Check sheet for the modelled part. Datum: model origin and axes. Units: mm. Give positions to 0.01 mm unless a question says otherwise; leave off trailing zeros. Loops run counter-clockwise (first coordinate to the right, second up) from the corner with the lowest first, then second, coordinate; pieces in that order, holes last. Notation, with made-up numbers: (78, 73.5) -> (127, 73.5) arc R5 ccw to (127, 80.5) -> close; hole circle Ø2 at (44, 33). An arc over 180 degrees is marked (long way). Write each question's results on one line, items separated by ' | '. Start each with the question number.
Item 1: Cross-section at D-D on z = 0.75. Enter the section's corners in (x, y), then the cut area to 3 significant figures.
Item 2: Mould release check, pull along X, two halves, no side actions. Record for faces 1 (the face through (17.5, 0, 0)), 2 (the face through (12.43, -3.905, 0.867)), 3 (the face through (-9.87, 1.6, 0.22)), 4 (the face through (1.09, -0.05, -4.88)): pulls with the +X half, pulls with the -X half, needs draft (parallel to the pull), parting line crosses it, or undercut.
Item 3: Cross-section at B-B on x = 15.25. Enter the section's corners in (y, z), then the cut area to 3 significant figures.
Item 4: Scan lines: line 1 along X through (y, z) = (-5, 0.5); line 2 along X through (y, z) = (7.5, 4); line 3 along Z through (x, y) = (2.5, 6.5). Record each from-to range of solid material in increasing order.
Item 5: Gauge pin test, flat ends, axial feed: pin 1 Ø12 at (x, z) = (8.5, -4) entering from +Y; pin 2 Ø2 at (y, z) = (8.5, 3.5) entering from +X; pin 3 Ø5 at (x, z) = (-7.5, 0) entering from -Y; pin 4 Ø12 at (y, z) = (6, 3.5) entering from +X. Record the tip position at first contact, or that the pin passes through.
Item 6: Cross-section at C-C on z = -5.5. Enter the section's corners in (x, y).
Item 7: Cross-section at A-A on z = -3. Enter the section's corners in (x, y).
from build123d import *

# Parameters (mm, degrees)
EXTRUDE_3_DEPTH      = 10
EXTRUDE_3_DEPTH_BACK = 10
SKETCH_3_R           = 5
CUT_EXTRUDE_1_DEPTH  = 27.477518989
EXTRUDE_6_DEPTH      = 10
EXTRUDE_6_DEPTH_BACK = 10
SKETCH_9_R           = 4
EXTRUDE_8_DEPTH      = 10


with BuildPart() as part:
    # Sketch 3D_4 → Extrude 3 (new, two sides: drawn at the far end of the back side and taken through both)
    with BuildSketch(Plane(origin=(0, 0, -10), x_dir=(0.24333901077648587, -0.042907233058801585, 0.9689917931466494), z_dir=(0.17364817766692725, 0.9848077530122086, 0)).offset(-EXTRUDE_3_DEPTH_BACK)):
        with BuildLine():
            Line((0, 0), (1.260173827, 4.941858145))
            Line((1.260173827, 4.941858145), (20.64000969, 0))
            Line((20.64000969, 0), (19.379835863, -4.941858145))
            ThreePointArc((19.379835863, -4.941858145), (7.218988859, -12.160847004), (0, 0))
        make_face()
    extrude(amount=EXTRUDE_3_DEPTH + EXTRUDE_3_DEPTH_BACK)

    # Sketch 3 → Cut-Extrude 1 (cut, through all)
    with BuildSketch(Plane(origin=(1.736481777, 9.84807753, 0), x_dir=(0.9848077530122086, -0.17364817766692736, 0), z_dir=(0.17364817766692736, 0.9848077530122086, 0))):
        with Locations(Location((0, 0, 0), (0, 0, 180))):
            Circle(SKETCH_3_R)
    extrude(amount=-CUT_EXTRUDE_1_DEPTH, mode=Mode.SUBTRACT)

    # Sketch 3D_9 → Extrude 6 (add, two sides: drawn at the far end of the back side and taken through both)
    with BuildSketch(Plane(origin=(7.5, 8.831813764, 0), x_dir=(0, -1, 0), z_dir=(0, 0, -1)).offset(-EXTRUDE_6_DEPTH_BACK)):
        Polygon((0, 0), (20.308532238, 0), (19.565497, 4.213962236), (-0.13065806, 0.740998683), align=None)
    extrude(amount=EXTRUDE_6_DEPTH + EXTRUDE_6_DEPTH_BACK)

    # Sketch 9 → Extrude 8 (add)
    with BuildSketch(Plane(origin=(7.5, 0, 0), x_dir=(0, 0, -1), z_dir=(1, 0, 0))):
        Circle(SKETCH_9_R)
    extrude(amount=EXTRUDE_8_DEPTH)


solid = part.part
Answer sheet:
1) outline: (-11.56, -8.12) -> (-6.6, -8.99) -> (-3.13, 10.71) -> (-8.08, 11.58) -> close; (3.13, -10.71) -> (7.5, -11.48) -> (7.5, -3.93) -> (17.5, -3.93) -> (17.5, 3.93) -> (7.5, 3.93) -> (7.5, 8.83) -> (6.6, 8.99) -> close | area: 233 mm²
2) face 1: pulls with the +X half | face 2: needs draft | face 3: pulls with the -X half | face 4: undercut
3) outline: circle Ø8 at (0, 0) | area: 50.3 mm²
4) line 1: x = -11.02 to -5.93, 4.17 to 7.5 | line 2: x = -7.98 to -1.72, 4.37 to 7.5 | line 3: z = -10 to -4.82, 4.82 to 10
5) pin 1: stops at y = 9.7 | pin 2: stops at x = 7.5 | pin 3: stops at y = -9.06 | pin 4: stops at x = 17.5
6) outline: (-9.96, -8.4) -> (7.5, -11.48) -> (7.5, 8.83) -> (-6.49, 11.3) -> close
7) outline: (-11.13, -8.19) -> (-5.68, -9.15) -> (-2.2, 10.54) -> (-7.66, 11.5) -> close; (2.2, -10.54) -> (7.5, -11.48) -> (7.5, -2.65) -> (17.5, -2.65) -> (17.5, 2.65) -> (7.5, 2.65) -> (7.5, 8.83) -> (5.68, 9.15) -> close
